```python
from build123d import *

# Parameters (mm, degrees)
BOSS_EXTRUDE1_DEPTH         = 32
SKETCH2_R                   = 9.5
CUT_EXTRUDE1_DEPTH          = 0.3
SKETCH3_R                   = 4
CUT_EXTRUDE2_DEPTH          = 5
CUT_EXTRUDE3_DEPTH          = 20
CUT_EXTRUDE4_DEPTH          = 76.531450403
CUT_EXTRUDE4_DEPTH_BACK     = 76.531450403
SKETCH5_R                   = 1.5
M3_TAPPED_HOLE1_D           = 2.5
M3_TAPPED_HOLE1_DEPTH       = 7.5
M3_TAPPED_HOLE1_CSINK_D     = 3.05
M3_TAPPED_HOLE1_CSINK_ANGLE = 90
M3_TAPPED_HOLE1_TIP         = 0.751075774
SKETCH9_W                   = 39.8
SKETCH9_H                   = 23.4
BOSS_EXTRUDE2_DEPTH         = 1.1
SKETCH10_R                  = 6
BOSS_EXTRUDE3_DEPTH         = 8.4
SKETCH11_R                  = 6
BOSS_EXTRUDE4_DEPTH         = 5
SKETCH12_R                  = 6.894871922
BOSS_EXTRUDE5_DEPTH         = 3.3
FILLET1_R                   = 2
M3_TAPPED_HOLE2_D           = 2.5
M3_TAPPED_HOLE2_DEPTH       = 7.5
M3_TAPPED_HOLE2_CSINK_D     = 3.05
M3_TAPPED_HOLE2_CSINK_ANGLE = 90
M3_TAPPED_HOLE2_TIP         = 0.751075774


with BuildPart() as part:
    # Sketch1 → Boss-Extrude1 (new body)
    with BuildSketch(Plane.XY):
        Polygon((-25.5, 51), (-25.5, 41), (0, 41), (0, 0), (-52, 0), (-52, 51), align=None)
    extrude(amount=BOSS_EXTRUDE1_DEPTH)

    # Sketch2 → Cut-Extrude1 (cut)
    with BuildSketch(Plane.ZY.offset(52)):
        with Locations((16, 16.75)):
            Circle(SKETCH2_R)
    extrude(amount=-CUT_EXTRUDE1_DEPTH, mode=Mode.SUBTRACT)

    # Sketch3 → Cut-Extrude2 (cut)
    with BuildSketch(Plane.ZY.offset(51.7)):
        with Locations((16, 16.75)):
            Circle(SKETCH3_R)
    extrude(amount=-CUT_EXTRUDE2_DEPTH, mode=Mode.SUBTRACT)

    # Sketch4 → Cut-Extrude3 (cut)
    with BuildSketch(Plane.XY.offset(32)):
        with BuildLine():
            Line((-6, 3), (-6, 0))
            Line((-6, 0), (0, 0))
            Line((0, 0), (0, 6))
            Line((0, 6), (-3, 6))
            ThreePointArc((-3, 6), (-5.121320344, 5.121320344), (-6, 3))
        make_face()
        with BuildLine():
            Line((-52, 45), (-49, 45))
            ThreePointArc((-49, 45), (-46.878679656, 45.878679656), (-46, 48))
            Line((-46, 48), (-46, 51))
            Line((-46, 51), (-52, 51))
            Line((-52, 51), (-52, 45))
        make_face()
    extrude(amount=-CUT_EXTRUDE3_DEPTH, mode=Mode.SUBTRACT)

    # Sketch5 → Cut-Extrude4 (cut, two sides: drawn at the far end of the back side and taken through both)
    with BuildSketch(Plane.XY.offset(12).offset(-CUT_EXTRUDE4_DEPTH_BACK)):
        with Locations((-3, 3)):
            Circle(SKETCH5_R)
        with Locations((-49, 48)):
            Circle(SKETCH5_R)
    extrude(amount=CUT_EXTRUDE4_DEPTH + CUT_EXTRUDE4_DEPTH_BACK, mode=Mode.SUBTRACT)

    # M3 Tapped Hole1
    with Locations(Plane(origin=(0, 0, 0), x_dir=(-1, 0, 0), z_dir=(0, 0, -1))):
        with Locations((7, 31), (7, 11), (47, 31)):
            CounterSinkHole(M3_TAPPED_HOLE1_D / 2, M3_TAPPED_HOLE1_CSINK_D / 2, depth=M3_TAPPED_HOLE1_DEPTH, counter_sink_angle=M3_TAPPED_HOLE1_CSINK_ANGLE)
            with Locations((0, 0, -(M3_TAPPED_HOLE1_DEPTH + M3_TAPPED_HOLE1_TIP / 2))):  # 118° drill point
                Cone(0, M3_TAPPED_HOLE1_D / 2, M3_TAPPED_HOLE1_TIP, mode=Mode.SUBTRACT)

    # Sketch9 → Boss-Extrude2 (add)
    with BuildSketch(Plane.XZ):
        with Locations((-28.3, 15.3)):
            Rectangle(SKETCH9_W, SKETCH9_H)
    extrude(amount=BOSS_EXTRUDE2_DEPTH)

    # Sketch10 → Boss-Extrude3 (add)
    with BuildSketch(Plane(origin=(0, 0, 0), x_dir=(0, 0, -1), z_dir=(1, 0, 0))):
        with Locations(Location((-16, 18.94541958, 0), (0, 0, 180))):
            Circle(SKETCH10_R)
    extrude(amount=BOSS_EXTRUDE3_DEPTH)

    # Sketch11 → Boss-Extrude4 (add)
    with BuildSketch(Plane(origin=(0, 51, 0), x_dir=(1, 0, 0), z_dir=(0, 1, 0))):
        with Locations(Location((-34, -16, 0), (0, 0, 90))):
            Circle(SKETCH11_R)
    extrude(amount=BOSS_EXTRUDE4_DEPTH)

    # Sketch12 → Boss-Extrude5 (add)
    with BuildSketch(Plane(origin=(0, 41, 0), x_dir=(1, 0, 0), z_dir=(0, 1, 0))):
        with Locations(Location((-18.5, -16, 0), (0, 0, 90))):
            Circle(SKETCH12_R)
    extrude(amount=BOSS_EXTRUDE5_DEPTH)

    # Fillet1
    # the kernel refuses this fillet: 2 mm, written as the material it adds along each edge
    with BuildSketch(Plane(origin=(-34, 51, 16), x_dir=(0, 0, -1), z_dir=(1, 0, 0))) as fillet1_piece_1:
        with BuildLine():
            CenterArc((6 + FILLET1_R, FILLET1_R), FILLET1_R, 180, 90)
            Line((6, FILLET1_R), (6, 0))
            Line((6, 0), (6 + FILLET1_R, 0))
        make_face()
    revolve(axis=Axis((-34, 51, 16), (0, 1, 0)))
    with BuildSketch(Plane(origin=(-18.5, 41, 16), x_dir=(0, 0, -1), z_dir=(1, 0, 0))) as fillet1_piece_2:
        with BuildLine():
            CenterArc((6.894871922 + FILLET1_R, FILLET1_R), FILLET1_R, 180, 90)
            Line((6.894871922, FILLET1_R), (6.894871922, 0))
            Line((6.894871922, 0), (6.894871922 + FILLET1_R, 0))
        make_face()
    revolve(axis=Axis((-18.5, 41, 16), (0, 1, 0)))
    with BuildSketch(Plane(origin=(0, 18.94541958, 16), x_dir=(0, 0, 1), z_dir=(0, 1, 0))) as fillet1_piece_3:
        with BuildLine():
            CenterArc((6 + FILLET1_R, FILLET1_R), FILLET1_R, 180, 90)
            Line((6, FILLET1_R), (6, 0))
            Line((6, 0), (6 + FILLET1_R, 0))
        make_face()
    revolve(axis=Axis((0, 18.94541958, 16), (1, 0, 0)))

    # M3 Tapped Hole2
    with Locations(Plane.XY.offset(32)):
        with Locations((-34, 46.5), (-18.5, 29.7), (-6, 17)):
            CounterSinkHole(M3_TAPPED_HOLE2_D / 2, M3_TAPPED_HOLE2_CSINK_D / 2, depth=M3_TAPPED_HOLE2_DEPTH, counter_sink_angle=M3_TAPPED_HOLE2_CSINK_ANGLE)
            with Locations((0, 0, -(M3_TAPPED_HOLE2_DEPTH + M3_TAPPED_HOLE2_TIP / 2))):  # 118° drill point
                Cone(0, M3_TAPPED_HOLE2_D / 2, M3_TAPPED_HOLE2_TIP, mode=Mode.SUBTRACT)


solid = part.part
```
Here's how the part is built. I have some questions about the finished solid (model axes, mm). A direction names the side the tool comes from. Round coordinates to 2 decimals unless told otherwise and drop trailing zeros. Use CSV: the item, a comma, the result in double quotes.
1) On a 3-axis mill with a long thin cutter (end or side, diameter ignored), from which of +Z, -Z, +X, -X, +Y, -Y can I reach the whole of each face in a straight line? I mean faces 1 (the cylindrical face through (-7.921, 31.845, 3.938)), 2 (the flat face through (-1, 6, 22)), 3 (the flat face through (-46.7, 17, 16)), 4 (the flat face through (-19, 44.3, 16)). Say none if no direction works.
Taken from the geometry:
face 1,"-Z"
face 2,"+Z, +X, -Y"
face 3,"-X"
face 4,"+Z, -Z, +X, +Y"
2) If we mould it in two halves opening along Z, with no side actions, what happens to faces 5 (the cylindrical face through (-33.84, 47.74, 28.06)), 6 (the cylindrical face through (-49.24, 19.45, 13.05)), 7 (the cylindrical face through (-25.336, 43.641, 16.898))? For each: pulls with the +Z half, pulls with the -Z half, needs draft (parallel to the pull), parting line crosses it, or undercut.
Taken from the geometry:
face 5,"needs draft"
face 6,"undercut"
face 7,"parting line crosses it"
3) I'm going to push flat-ended pins straight in: P1, Ø8, axis at y = 44, z = 17, coming from the +X side; P2, Ø1.5, axis at x = -1, z = 18, coming from the -Y side; P3, Ø0.9, axis at x = -51, z = 17.5, coming from the +Y side. Where does each tip first touch, or does it pass through?
Taken from the geometry:
P1,"x = 0"
P2,"y = 6"
P3,"y = 45"
4) I need wall thicknesses on line 1 along Y through (x, z) = (-7, 4.75); line 2 along X through (y, z) = (29.7, 28.75); line 3 along X through (y, z) = (31, 6). Which ranges of each line are inside material? Lowest first, please. Write a range as [from, to].
Taken from the geometry:
line 1,"[0, 9.75], [12.25, 29.75], [32.25, 41]"
line 2,"[-52, -19.75], [-17.25, 0]"
line 3,"[-52, -48.25], [-45.75, -8.25], [-5.75, 0]"
